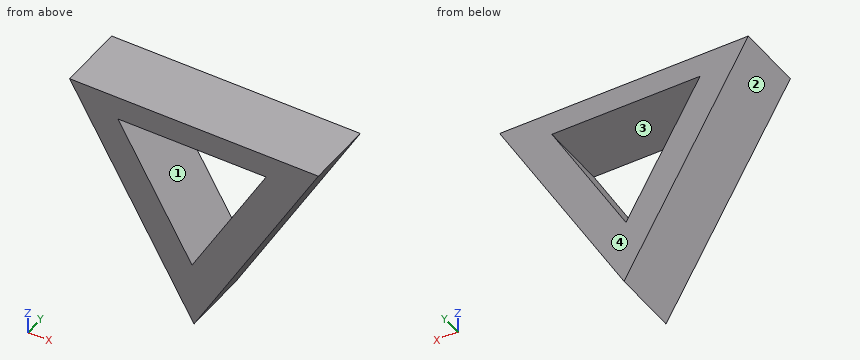
from build123d import *

# Parameters (mm, degrees)
F1_DEPTH = 25.4


with BuildPart() as f1:
    # F0 (on Front) → F1 (new body)
    with BuildSketch(Plane.XZ):
        Polygon((-46.694561, 80.877353), (0, 0), (46.694561, 80.877353), align=None)
        Polygon((-0.743479, 23.911752), (-28.570018, 72.108731), (27.08306, 72.108731), align=None, mode=Mode.SUBTRACT)
    extrude(amount=F1_DEPTH)


solid = f1.part
Build history of the part. All positions in model axes, mm. Face numbers are marked on the shaded views. Coordinates: 2 decimals unless noted, no trailing zeros. Order: outer loops, then holes, each group sorted by start corner. A loop starts at its lowest first (then second) coordinate and runs counter-clockwise, first axis right, second up. Notation, with made-up numbers: M 4.25,32.5 L 57.25,32.5 A22 cw 57.25,69.5 Z; hole C 88,-4 d2. An arc over 180 degrees is marked long. One line per question, with ' | ' between items. Start each with the question number.
Q1. Two-plate mould, pull along X, no slides. Class the marked faces 1, 2, 3 and 4: +X half, -X half, draft (parallel to the pull), parting line (faces both ways), or undercut.
Q2. Saw through at D-D (z = 7). List the corners of the cut face in (x, y), then the cut area to 3 significant figures.
Q3. Saw through at A-A (z = 47). List the corners of the cut face in (x, y).
Q4. Probe L1, parallel to Z at x = -23, y = -17.25; L2, parallel to Z at x = 1.5, y = -12.5; L3, parallel to X at y = -3, z = 60.5. List the from-to ranges inside material, lowest first. Write a range as from..to.
Q5. Flat gauge pins, fed straight in: pin 1 Ø5 at (y, z) = (-15, 53.5) entering from +X; pin 2 Ø6 at (y, z) = (-7.5, 48.5) entering from -X; pin 3 Ø8 at (x, y) = (32.5, -22.5) entering from -Z. Where does each tip first touch, or does it go through?
Q6. Saw through at B-B (x = -3). List the corners of the cut face in (y, z), then the cut area to 3 significant figures.
Q7. Saw through at C-C (y = -9.5). List the corners of the cut face in (x, z), then the cut area to 3 significant figures.
Check values:
1) face 1: undercut | face 2: -X half | face 3: undercut | face 4: draft
2) outline: M -4.04,-25.4 L 4.04,-25.4 L 4.04,0 L -4.04,0 Z | area: 205 mm2
3) outline: M -27.14,-25.4 L -14.07,-25.4 L -14.07,0 L -27.14,0 Z; M 12.59,-25.4 L 27.14,-25.4 L 27.14,0 L 12.59,0 Z
4) L1: z = 39.84..62.46, 72.11..80.88 | L2: z = 2.6..27.8, 72.11..80.88 | L3: x = -34.93..-21.87, 20.38..34.93
5) pin 1: stops at x = 32.33 | pin 2: stops at x = -29.73 | pin 3: stops at z = 49.36
6) outline: M -25.4,5.2 L 0,5.2 L 0,27.82 L -25.4,27.82 Z; M -25.4,72.11 L 0,72.11 L 0,80.88 L -25.4,80.88 Z | area: 797 mm2
7) outline: M -46.69,80.88 L 0,0 L 46.69,80.88 Z; hole M -28.57,72.11 L -0.74,23.91 L 27.08,72.11 Z | area: 2,440 mm2
